Verification items for this drawing (mm, ordinates from the low corner). A direction names the side the tool comes from. Round coordinates to 2 decimals unless told otherwise and drop trailing zeros. Order: outer loops, then holes, each group sorted by start corner. A loop starts at its lowest first (then second) coordinate and runs counter-clockwise, first axis right, second up. Notation, with made-up numbers: (18, -27) -> (64, -27) arc R34 ccw to (64, 5) -> close; hole circle Ø10 at (39.5, 16.5). An arc over 180 degrees is marked (long way). Put each result on its own line as item: value.
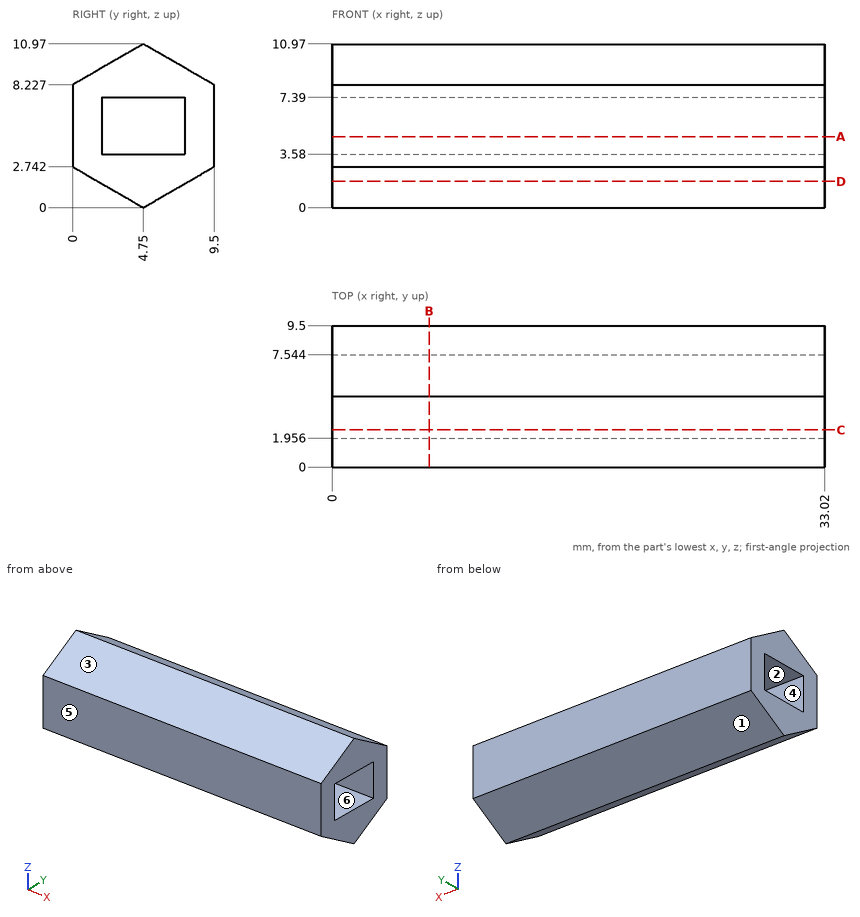
Item 1: Section check A-A on z = 4.75. Record the boundary of the cut face in (x, y).
Check sheet entries:
outline: (0, 0) -> (33.02, 0) -> (33.02, 1.96) -> (0, 1.96) -> close; (0, 7.54) -> (33.02, 7.54) -> (33.02, 9.5) -> (0, 9.5) -> close
Item 2: Section check C-C on y = 2.5. Record the boundary of the cut face in (x, z).
Check sheet entries:
outline: (0, 1.3) -> (33.02, 1.3) -> (33.02, 3.58) -> (0, 3.58) -> close; (0, 7.39) -> (33.02, 7.39) -> (33.02, 9.67) -> (0, 9.67) -> close
Item 3: Section check B-B on x = 6.5. Record the boundary of the cut face in (y, z).
Check sheet entries:
outline: (0, 2.74) -> (4.75, 0) -> (9.5, 2.74) -> (9.5, 8.23) -> (4.75, 10.97) -> (0, 8.23) -> close; hole (1.96, 3.58) -> (7.54, 3.58) -> (7.54, 7.39) -> (1.96, 7.39) -> close
Item 4: Section check D-D on z = 1.75. Record the boundary of the cut face in (x, y), then the cut area to 3 significant figures.
Check sheet entries:
outline: (0, 1.72) -> (33.02, 1.72) -> (33.02, 7.78) -> (0, 7.78) -> close
area: 200 mm^2
Item 5: Tool access check on the marked faces 1 and 2. Record the directions out of +Z, -Z, +X, -X, +Y, -Y that give a thin tool (end or side, any length) a straight path to the whole face; none if there is none.
Check sheet entries:
face 1: -Z, +X, -X, +Y
face 2: +X, -X
Item 6: Gauge pin test, flat ends, axial feed: pin 1 Ø1 at (x, z) = (18, 2.5) entering from +Y; pin 2 Ø3 at (x, z) = (8.5, 10) entering from +Y (1 decimal); pin 3 Ø4.5 at (x, y) = (21, 4.5) entering from -Z. Record the tip position at first contact, or that the pin passes through.
Check sheet entries:
pin 1: stops at y = 9.5
pin 2: stops at y = 9
pin 3: stops at z = 0
Item 7: Release check for a two-part mould opening along Z. For the marked faces 3, 4, 5 and 6 record: +Z half, -Z half, draft (parallel to the pull), parting line (faces both ways), or undercut.
Check sheet entries:
face 3: +Z half
face 4: undercut
face 5: draft
face 6: undercut
Item 8: Material ranges on L1, parallel to Y at x = 14.5, z = 6; L2, parallel to Z at x = 12, y = 6; L3, parallel to Z at x = 8.5, y = 4.5 (1 decimal), recorded low to high. Write a range as [from, to].
Check sheet entries:
L1: y = [0, 1.96], [7.54, 9.5]
L2: z = [0.72, 3.58], [7.39, 10.25]
L3: z = [0.1, 3.6], [7.4, 10.8]
